Work out the finished part from the listing and answer in its coordinate system (mm). A direction names the side the tool comes from. Give positions to 0.01 mm unless a question says otherwise; leave off trailing zeros. Order: outer loops, then holes, each group sorted by start corner. A loop starts at its lowest first (then second) coordinate and runs counter-clockwise, first axis right, second up.
Autodesk Inventor part; units mm, degrees
ref_plane "YZ Plane" through (0, 0, 0) normal (1, 0, 0) x (0, 1, 0)
ref_plane "XZ Plane" through (0, 0, 0) normal (0, 1, 0) x (-1, 0, 0)
ref_plane "XY Plane" through (0, 0, 0) normal (0, 0, 1) x (1, 0, 0)
sketch "Sketch1" plane through (0, 0, 0) normal (0, 0, 1) x (1, 0, 0)
  line L0 (0, 0) -> (4, 0)
  line L1 (4, 0) -> (4, 5)
  line L2 (4, 5) -> (0, 5)
  line L3 (0, 5) -> (0, 0)
  point P0 (0, 2.5)
  dimension "d0" = 5
  dimension "d1" = 8
revolve "Revolution1" add sketch "Sketch1" angle 360 about axis through (0, 5, 0) along (0, -1, 0)
sketch "Sketch2" plane through (0, 5, 0) normal (0, 1, 0) x (1, 0, 0)
  circle A0 centre (0, 0) radius 4
  circle A1 centre (0, 0) radius 4
  line L0 (-3.9291, -0.75) -> (3.9291, -0.75)
  line L1 (-3.9291, 0.75) -> (3.9291, 0.75)
  point P0 (0, -0.75)
  dimension "d3" = 0.75
  dimension "d4" = 0.75
extrude "Extrusion1" cut sketch "Sketch2" against normal blind 1 contours A0 L0 L1
sketch "Sketch3" plane through (0, 0, 0) normal (0, -1, 0) x (1, 0, 0)
  circle A0 centre (0, 0) radius 4
hole "Hole1" at (0, 0, 0) direction (0, 1, 0) diameter 6 depth 1.5
thread "Thread1"
properties part number "138"
1. The mould has two halves that part along Z. Classify faces 1 (the face through (0, 5, -2)), 2 (the face through (3.695, 2.535, 1.532)), 3 (the face through (0, 4, 0)): pulls with the +Z half, pulls with the -Z half, needs draft (parallel to the pull), parting line crosses it, or undercut.
Findings below:
face 1: needs draft
face 2: parting line crosses it
face 3: undercut
2. Which of the six approach directions +Z, -Z, +X, -X, +Y, -Y give full straight-line access (tool end or side, diameter ignored) to faces 4 (the face through (-0.1, 4.5, -0.75)), 5 (the face through (0, 1.5, 0)), 6 (the face through (0, 5, 2))?
Findings below:
face 4: +X, -X, +Y
face 5: -Y
face 6: +Z, -Z, +X, -X, +Y
3. The part is cut by section B-B (x = 0). Write down the section's boundary in (y, z).
Findings below:
outline: (0, -4) - (5, -4) - (5, -0.75) - (4, -0.75) - (4, 0.75) - (5, 0.75) - (5, 4) - (0, 4) - (0, 3) - (1.5, 3) - (1.5, -3) - (0, -3) - close
4. Given P1, Ø1, axis at y = 3.5, z = -2.5, coming from the +X side; P2, Ø1.5, axis at x = 3, y = 1, coming from the +Z side; P3, Ø1.1, axis at x = 1.5, y = 4.5, coming from the +Z side, each flat-ended and moving along its own axis, determine where each tip first touches the part or whether it passes through.
Findings below:
P1: stops at x = 3.46
P2: stops at z = 3.31
P3: stops at z = 3.89
5. The part is cut by section C-C (y = 0.3). Write down the section's boundary in (x, z).
Findings below:
outline: circle Ø8 at (0, 0); hole circle Ø6 at (0, 0)
6. Straight lines are drawn through the part: probe 1 along X at (y, z) = (0.55, 0); probe 2 along Y at (x, z) = (1.5, 0.5). For each, find the intervals that lie inside material, in ascending order.
Findings below:
probe 1: x = -4 to -3, 3 to 4
probe 2: y = 1.5 to 4
7. The part is cut by section A-A (z = 0). Write down the section's boundary in (x, y), then the cut area to 3 significant figures.
Findings below:
outline: (-4, 0) - (-3, 0) - (-3, 1.5) - (3, 1.5) - (3, 0) - (4, 0) - (4, 4) - (-4, 4) - close
area: 23.0 mm2
8. The part is cut by section D-D (y = 2.1). Write down the section's boundary in (x, z).
Findings below:
outline: circle Ø8 at (0, 0)
